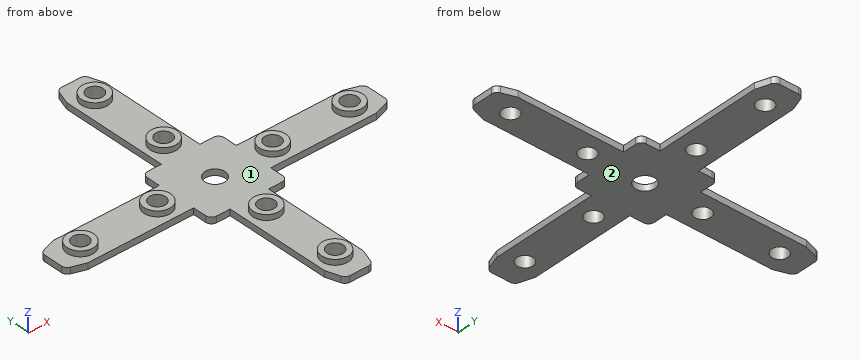
```python
from build123d import *

# Parameters (mm, degrees)
SKETCH1_R             = 2.6
BOSS_EXTRUDE1_DEPTH   = 1.6
SKETCH2_R             = 3.45
BOSS_EXTRUDE2_DEPTH   = 1.4
M5X0_8_TAPPED_HOLE1_D = 4.2


with BuildPart() as part:
    # Sketch1 → Boss-Extrude1 (new body)
    with BuildSketch(Plane.XY):
        with BuildLine():
            Line((-10, -8.5), (-10, -5))
            Line((-10, -5), (-37.5, -5))
            Line((-37.5, -5), (-40.974341649, -3.841886117))
            ThreePointArc((-40.974341649, -3.841886117), (-41.716863278, -3.295926597), (-42, -2.41886117))
            Line((-42, -2.41886117), (-42, 2.41886117))
            ThreePointArc((-42, 2.41886117), (-41.716863278, 3.295926597), (-40.974341649, 3.841886117))
            Line((-40.974341649, 3.841886117), (-37.5, 5))
            Line((-37.5, 5), (-10, 5))
            Line((-10, 5), (-10, 8.5))
            ThreePointArc((-10, 8.5), (-9.560660172, 9.560660172), (-8.5, 10))
            Line((-8.5, 10), (-5, 10))
            Line((-5, 10), (-5, 37.485))
            Line((-5, 37.485), (-3.841886117, 40.959341649))
            ThreePointArc((-3.841886117, 40.959341649), (-3.295926597, 41.701863278), (-2.41886117, 41.985))
            Line((-2.41886117, 41.985), (2.41886117, 41.985))
            ThreePointArc((2.41886117, 41.985), (3.295926597, 41.701863278), (3.841886117, 40.959341649))
            Line((3.841886117, 40.959341649), (5, 37.485))
            Line((5, 37.485), (5, 10))
            Line((5, 10), (8.5, 10))
            ThreePointArc((8.5, 10), (9.560660172, 9.560660172), (10, 8.5))
            Line((10, 8.5), (10, 5))
            Line((10, 5), (37.5, 5))
            Line((37.5, 5), (40.974341649, 3.841886117))
            ThreePointArc((40.974341649, 3.841886117), (41.716863278, 3.295926597), (42, 2.41886117))
            Line((42, 2.41886117), (42, -2.41886117))
            ThreePointArc((42, -2.41886117), (41.716863278, -3.295926597), (40.974341649, -3.841886117))
            Line((40.974341649, -3.841886117), (37.5, -5))
            Line((37.5, -5), (10, -5))
            Line((10, -5), (10, -8.5))
            ThreePointArc((10, -8.5), (9.560660172, -9.560660172), (8.5, -10))
            Line((8.5, -10), (5, -10))
            Line((5, -10), (5, -37.485))
            Line((5, -37.485), (3.841886117, -40.959341649))
            ThreePointArc((3.841886117, -40.959341649), (3.295926597, -41.701863278), (2.41886117, -41.985))
            Line((2.41886117, -41.985), (-2.41886117, -41.985))
            ThreePointArc((-2.41886117, -41.985), (-3.295926597, -41.701863278), (-3.841886117, -40.959341649))
            Line((-3.841886117, -40.959341649), (-5, -37.485))
            Line((-5, -37.485), (-5, -10))
            Line((-5, -10), (-8.5, -10))
            ThreePointArc((-8.5, -10), (-9.560660172, -9.560660172), (-10, -8.5))
        make_face()
        Circle(SKETCH1_R, mode=Mode.SUBTRACT)
    extrude(amount=BOSS_EXTRUDE1_DEPTH)

    # Sketch2 → Boss-Extrude2 (add)
    with BuildSketch(Plane.XY.offset(1.6)):
        with Locations((0, 14.95)):
            Circle(SKETCH2_R)
        with Locations((0, 34.95)):
            Circle(SKETCH2_R)
        with Locations((0, -14.95)):
            Circle(SKETCH2_R)
        with Locations((0, -34.95)):
            Circle(SKETCH2_R)
        with Locations((-14.95, 0)):
            Circle(SKETCH2_R)
        with Locations((-34.95, 0)):
            Circle(SKETCH2_R)
        with Locations((14.95, 0)):
            Circle(SKETCH2_R)
        with Locations((34.95, 0)):
            Circle(SKETCH2_R)
    extrude(amount=BOSS_EXTRUDE2_DEPTH)

    # M5x0.8 Tapped Hole1 (through all)
    with Locations(Plane.XY.offset(3)):
        with Locations((0, 34.95), (0, 14.95), (0, -14.95), (0, -34.95), (-14.95, 0), (-34.95, 0), (14.95, 0), (34.95, 0)):
            Hole(M5X0_8_TAPPED_HOLE1_D / 2)


solid = part.part
```
Model file for the job. Use its own axes, mm. Face numbers are marked on the shaded views. Coordinates: 2 decimals unless noted, no trailing zeros. Write each loop counter-clockwise with the first axis right and the second up, starting at its lowest first coordinate (ties: lowest second). Pieces come first, ordered by that corner, then holes. Notation, with made-up numbers: (-32, -11.5) - (-2, -11.5) arc R18 cw to (-2, -1.5) - close; hole circle Ø5 at (9.5, -33.75). An arc over 180 degrees is marked (long way). One line per item, written item: value. Start each with the question number.
1. Probe line 1 (Y direction, x = 0, z = 1.25) (3 decimals); line 2 (Y direction, x = -14.95, z = 0.8); line 3 (Y direction, x = 15.5, z = 2.85). List the from-to ranges inside material, lowest first. Write a range as from..to.
2. Slice it at B-B (x = 34.95). Write the cut outline in (y, z), plus the area to 3 significant figures.
3. Slice it at A-A (z = 2.3). Count the separate pieces of the cut face and the enclosed holes in it, plus the area to 3 significant figures.
4. Mould opens along X. For the marked faces 1 and 2 say: released by +X, released by -X, zero draft, split by the parting line, or undercut.
5. Flat gauge pins, fed straight in: pin 1 (5.5 mm diameter, centred on x = -14.95, y = 0, fed in from -Z); pin 2 (0.8 mm diameter, centred on y = -7, z = 1, fed in from -X); pin 3 (1.3 mm diameter, centred on x = 22.5, z = 0.5, fed in from +Y); pin 4 (1.3 mm diameter, centred on y = 22, z = 0.5, fed in from +X). Where does each tip first touch, or does it go through?
Answers below:
1. line 1: y = -41.985..-37.05, -32.85..-17.05, -12.85..-2.6, 2.6..12.85, 17.05..32.85, 37.05..41.985
1. line 2: y = -5..-2.1, 2.1..5
1. line 3: y = -3.41..-2.03, 2.03..3.41
2. outline: (-5, 0) - (-2.1, 0) - (-2.1, 3) - (-3.45, 3) - (-3.45, 1.6) - (-5, 1.6) - close; (2.1, 0) - (5, 0) - (5, 1.6) - (3.45, 1.6) - (3.45, 3) - (2.1, 3) - close
2. area: 13.1 mm^2
3. separate pieces: 8
3. enclosed holes: 8
3. area: 188 mm^2
4. face 1: undercut
4. face 2: zero draft
5. pin 1: stops at z = 0
5. pin 2: stops at x = -10
5. pin 3: stops at y = 5
5. pin 4: stops at x = 5
